Answer from the drawing. Dimensions are ordinates in mm from the lowest x, y and z of the part. A direction names the side the tool comes from. Give positions to 0.01 mm unless a question says otherwise; leave off trailing zeros. Loops run counter-clockwise (first coordinate to the right, second up) from the corner with the lowest first, then second, coordinate; pieces in that order, holes last.
(1) Find section C-C, the plane y = 57.5. Write down the section's boundary in (x, z), then the cut area to 3 significant figures.
(2) Find section D-D, the plane x = 13. Write down the section's boundary in (y, z), then the cut area to 3 significant figures.
(3) Each of these flat-tipped pins is pushed along its axis until it touches: P1, Ø6, axis at x = 10, y = 55, coming from the +Z side; P2, Ø7.5, axis at x = 9, z = 36, coming from the +Y side; P3, Ø7, axis at x = 7.5, y = 58.48, coming from the -Z side. Where does it stop, or does it pass through?
(4) Find section B-B, the plane z = 7.5. Write down the section's boundary in (x, y), then the cut area to 3 significant figures.
(5) Straight lines are drawn through the part: probe 1 along Z at (x, y) = (7.5, 2.25); probe 2 along Y at (x, z) = (7.75, 16.5) (1 decimal); probe 3 along Z at (x, y) = (4.75, 59). For each, find the intervals that lie inside material, in ascending order.
(6) Find section A-A, the plane y = 50. Write down the section's boundary in (x, z).
(7) Determine the mould class of the marked faces 4, 5 and 6 for opening direction X: pulls with the +X half, pulls with the -X half, needs draft (parallel to the pull), parting line crosses it, or undercut.
(8) Which of the six approach directions +Z, -Z, +X, -X, +Y, -Y give full straight-line access (tool end or side, diameter ignored) to the marked faces 1, 2 and 3?
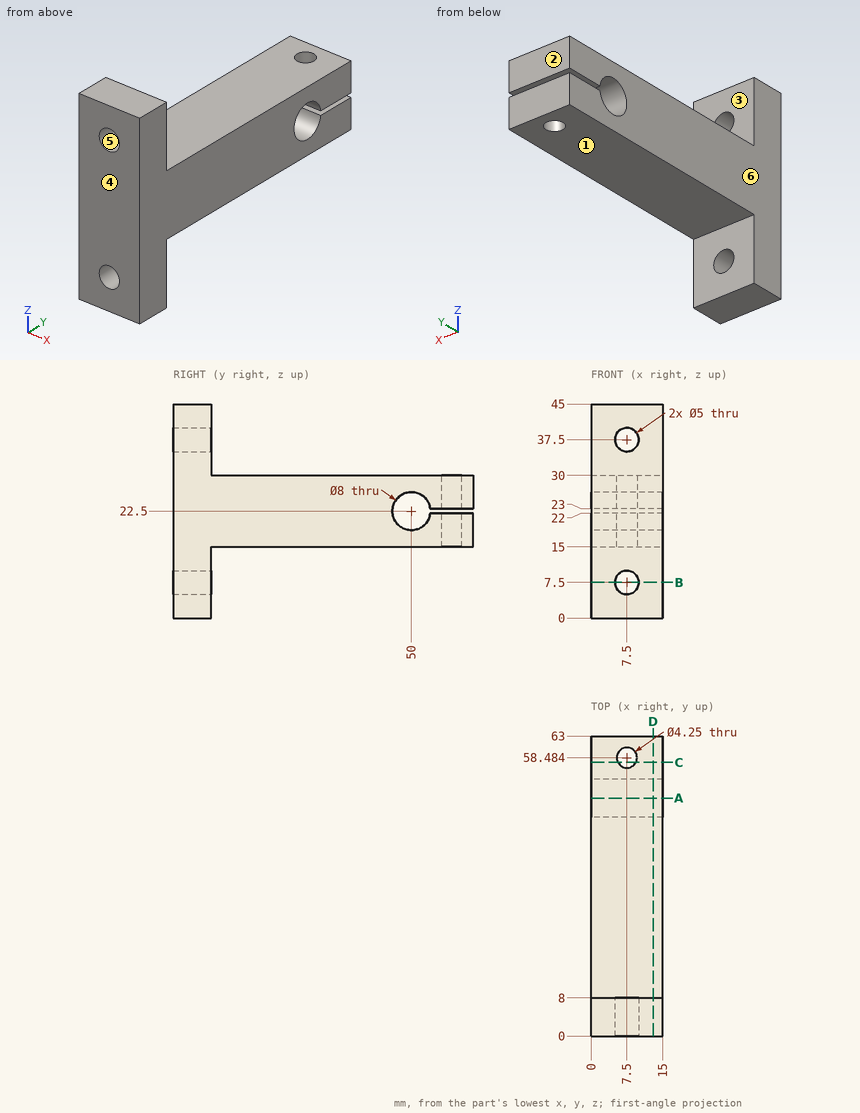
Entries:
1. outline: (0, 15) - (5.62, 15) - (5.62, 22) - (0, 22) - close; (0, 23) - (5.62, 23) - (5.62, 30) - (0, 30) - close; (9.38, 15) - (15, 15) - (15, 22) - (9.38, 22) - close; (9.38, 23) - (15, 23) - (15, 30) - (9.38, 30) - close
1. area: 157 mm2
2. outline: (0, 0) - (8, 0) - (8, 15) - (63, 15) - (63, 22) - (53.97, 22) arc R4 cw (long way) to (53.97, 23) - (63, 23) - (63, 30) - (8, 30) - (8, 45) - (0, 45) - close
2. area: 1,130 mm2
3. P1: stops at z = 30
3. P2: stops at y = 8
3. P3: stops at z = 15
4. outline: (0, 0) - (5, 0) - (5, 8) - (0, 8) - close; (10, 0) - (15, 0) - (15, 8) - (10, 8) - close
4. area: 80.0 mm2
5. probe 1: z = 0 to 5, 10 to 35, 40 to 45
5. probe 2: y = 0 to 56.4, 60.6 to 63
5. probe 3: z = 15 to 22, 23 to 30
6. outline: (0, 15) - (15, 15) - (15, 18.5) - (0, 18.5) - close; (0, 26.5) - (15, 26.5) - (15, 30) - (0, 30) - close
7. face 4: needs draft
7. face 5: undercut
7. face 6: pulls with the -X half
8. face 1: -Z, +X, -X, +Y
8. face 2: +Z, -Z, +X, -X, +Y
8. face 3: +Z, +X, -X, +Y
